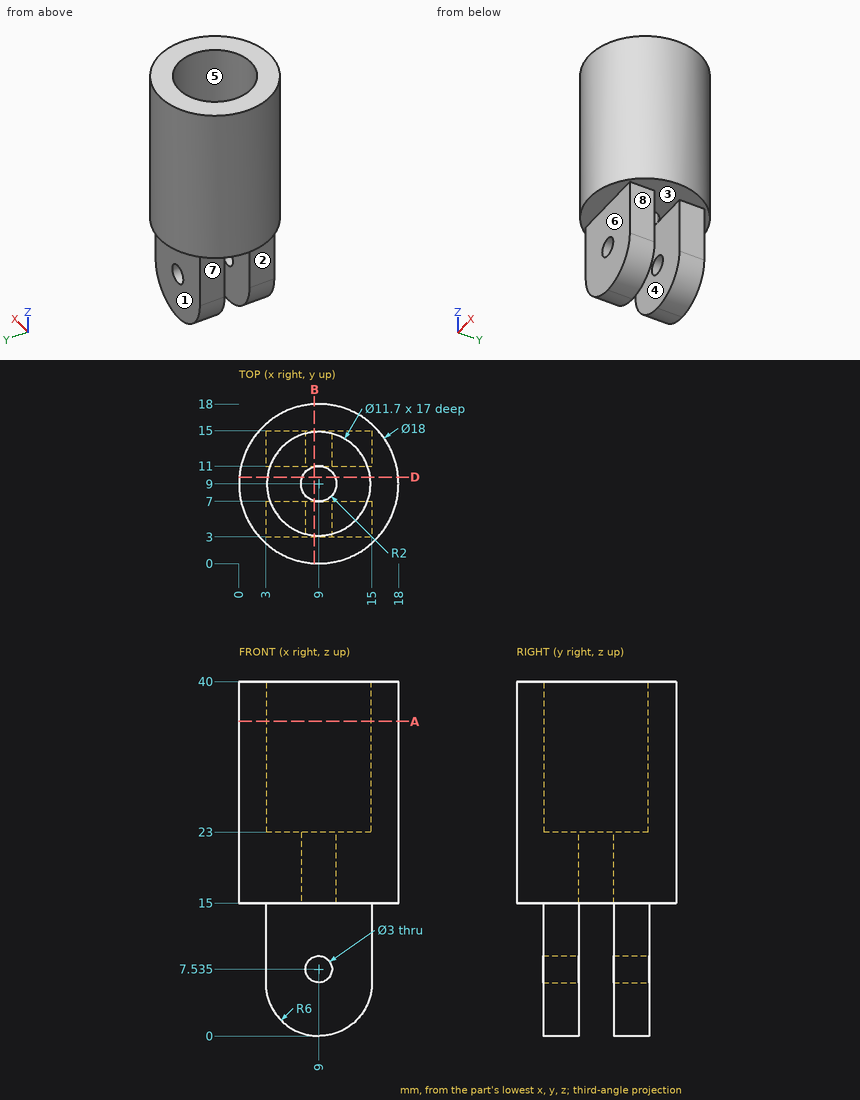
The figure shows three views and two pictorial views of one solid part (mm, origin at its lowest corner). Answer the questions. A direction names the side the tool comes from. Give positions to 0.01 mm unless a question says otherwise; leave off trailing zeros. Order: outer loops, then holes, each group sorted by start corner. A loop starts at its lowest first (then second) coordinate and runs counter-clockwise, first axis right, second up. Notation, with made-up numbers: (65, 0) -> (99, 0) arc R27 cw to (99, 18) -> close; hole circle Ø6 at (-28, -39.75). An arc over 180 degrees is marked (long way). One line per item, written item: value.
1) Find section D-D, the plane y = 9.75. Determine the outline of the cut face in (x, z), plus the area to 4 significant figures.
Reported:
outline: (0.03, 15) -> (7.15, 15) -> (7.15, 23) -> (3.2, 23) -> (3.2, 40) -> (0.03, 40) -> close; (10.85, 15) -> (17.97, 15) -> (17.97, 40) -> (14.8, 40) -> (14.8, 23) -> (10.85, 23) -> close
area: 221.5 mm^2
2) Flat-ended cylindrical pins translate along their axes: P1, Ø1.2, axis at y = 12.5, z = 10, coming from the +X side; P2, Ø3, axis at y = 6, z = 11.5, coming from the -X side; P3, Ø3.5, axis at x = 8, z = 5, coming from the -Y side; P4, Ø5, axis at x = 6.5, z = 25.5, coming from the -Y side. Find the tip coordinate at first contact, or state that the pin passes through.
Reported:
P1: stops at x = 15
P2: stops at x = 3
P3: stops at y = 3
P4: stops at y = 0
3) Find section B-B, the plane x = 8.5. Determine the outline of the cut face in (y, z), plus the area to 3 significant figures.
Reported:
outline: (0.01, 15) -> (3, 15) -> (3, 8.95) -> (7, 8.95) -> (7, 15) -> (7.06, 15) -> (7.06, 23) -> (3.17, 23) -> (3.17, 40) -> (0.01, 40) -> close; (3, 0.02) -> (7, 0.02) -> (7, 6.12) -> (3, 6.12) -> close; (10.94, 15) -> (11, 15) -> (11, 8.95) -> (15, 8.95) -> (15, 15) -> (17.99, 15) -> (17.99, 40) -> (14.83, 40) -> (14.83, 23) -> (10.94, 23) -> close; (11, 0.02) -> (15, 0.02) -> (15, 6.12) -> (11, 6.12) -> close
area: 317 mm^2
4) A tool of negligible diameter and unlimited length cuts with its end or side. For the marked faces 4, 5, 6, 7 and 8, from which of +Z, -Z, +X, -X, +Y, -Y can it reach the whole face along a straight path? Write none if from no direction.
Reported:
face 4: -Z, +X, -X
face 5: +Z
face 6: -Z, +X, -X, -Y
face 7: -Z, -X, +Y, -Y
face 8: -Z, +X, +Y, -Y
5) Find section A-A, the plane z = 35.5. Determine the outline of the cut face in (x, y), plus the area to 3 significant figures.
Reported:
outline: circle Ø18 at (9, 9); hole circle Ø11.7 at (9, 9)
area: 147 mm^2
6) Find the intervals of material crossed by line 1 (Y direction, x = 9, z = 34.5); line 2 (Z direction, x = 9, y = 3.95) (3 decimals); line 3 (Y direction, x = 14, z = 4), in increasing order.
Reported:
line 1: y = 0 to 3.15, 14.85 to 18
line 2: z = 0 to 6.035, 9.035 to 23
line 3: y = 3 to 7, 11 to 15
7) Determine the mould class of the marked faces 1, 2 and 3 for opening direction Y: pulls with the +Y half, pulls with the -Y half, needs draft (parallel to the pull), parting line crosses it, or undercut.
Reported:
face 1: pulls with the +Y half
face 2: needs draft
face 3: undercut
